```python
from build123d import *

# Parameters (mm, degrees)
BOSS_EXTRUDE1_DEPTH = 6.35
SKETCH2_R           = 2.8575
SKETCH2_W           = 7.62
SKETCH2_H           = 6.5024
SKETCH2_W_2         = 13.97
SKETCH2_H_2         = 3.81
CUT_EXTRUDE1_DEPTH  = 7.35
SKETCH3_W           = 5.334
SKETCH3_H           = 5.08
CUT_EXTRUDE2_DEPTH  = 13.97
SKETCH4_W           = 24.13
SKETCH4_H           = 11.681664872
CUT_EXTRUDE3_DEPTH  = 2.54
FILLET1_R           = 1.5875


with BuildPart() as part:
    # Sketch1 → Boss-Extrude1 (new body)
    with BuildSketch(Plane(origin=(0, 0, 0), x_dir=(0, 0, -1), z_dir=(1, 0, 0))):
        with BuildLine():
            Line((0, 2.54), (0, 14.474335183))
            Line((0, 14.474335183), (38.205942443, 14.474335183))
            ThreePointArc((38.205942443, 14.474335183), (39.475942443, 14.134039708), (40.405646968, 13.204335183))
            Line((40.405646968, 13.204335183), (41.796677285, 10.795))
            ThreePointArc((41.796677285, 10.795), (42.72638181, 9.865295474), (43.99638181, 9.525))
            Line((43.99638181, 9.525), (70.840761314, 9.525))
            Line((70.840761314, 9.525), (66.074734842, 1.27))
            ThreePointArc((66.074734842, 1.27), (65.145030316, 0.340295474), (63.875030316, 0))
            Line((63.875030316, 0), (2.54, 0))
            ThreePointArc((2.54, 0), (0.743948776, 0.743948776), (0, 2.54))
        make_face()
    extrude(amount=BOSS_EXTRUDE1_DEPTH)

    # Sketch2 → Cut-Extrude1 (cut, through all)
    with BuildSketch(Plane(origin=(6.35, 0, 0), x_dir=(0, 0, -1), z_dir=(1, 0, 0))):
        with Locations((59.69, 4.7625)):
            Circle(SKETCH2_R)
        with Locations((46.355, 4.7625)):
            Rectangle(SKETCH2_W, SKETCH2_H)
        with Locations((22.3393, 1.905)):
            Rectangle(SKETCH2_W_2, SKETCH2_H_2)
    extrude(amount=-CUT_EXTRUDE1_DEPTH, mode=Mode.SUBTRACT)

    # Sketch3 → Cut-Extrude2 (cut)
    with BuildSketch(Plane.XY.offset(-29.3243)):
        with Locations((2.667, 6.35)):
            Rectangle(SKETCH3_W, SKETCH3_H)
    extrude(amount=CUT_EXTRUDE2_DEPTH, mode=Mode.SUBTRACT)

    # Sketch4 → Cut-Extrude3 (cut)
    with BuildSketch(Plane(origin=(0, 0, 0), x_dir=(0, 0, -1), z_dir=(1, 0, 0))):
        with Locations((21.0693, 5.840832436)):
            Rectangle(SKETCH4_W, SKETCH4_H)
    extrude(amount=CUT_EXTRUDE3_DEPTH, mode=Mode.SUBTRACT)

    # Fillet1
    fillet1_edges = [part.edges().sort_by_distance(p)[0] for p in [
        (2.54, 8.89, -22.3393),
        (2.54, 4.445, -15.3543),
        (2.54, 4.445, -29.3243),
        (0, 5.840832436, -9.0043),
        (0, 5.840832436, -33.1343),
        (0, 11.681664872, -21.0693),
    ]]
    fillet(fillet1_edges, radius=FILLET1_R)


solid = part.part
```
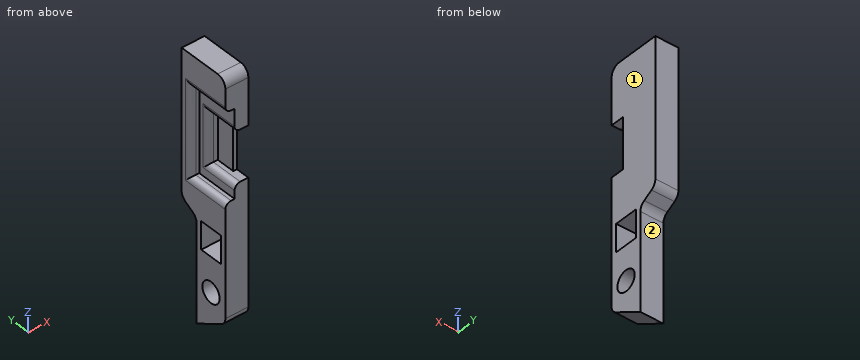
Geometry: final body of the model. Coordinates: model frame, mm. Face numbers are marked on the shaded views. A direction names the side the tool comes from. Coordinates: 2 decimals unless noted, no trailing zeros. Write each loop counter-clockwise with the first axis right and the second up, starting at its lowest first coordinate (ties: lowest second). Pieces come first, ordered by that corner, then holes. Notation, with made-up numbers: M -10.5,74 L -4.5,74 A21 cw -4.5,98 Z; hole C -25,-6 d5. An arc over 180 degrees is marked long. Answer as CSV lines item,"result". Start each with the question number.
Q1. Cut plane C-C on y = 6.25. Count the separate pieces of the cut face and the enclosed holes in it, then the cut area to 3 significant figures.
Q2. Reachability of the marked faces 1 and 2 from +Z, -Z, +X, -X, +Y, -Y: full face, straight path, thin tool, end or side. Return the list, or none.
Q3. Line query: line 1 (Y direction, x = 2.75, z = -59.69) (3 decimals); line 2 (Y direction, x = 1.5, z = -44) (3 decimals); line 3 (Z direction, x = 0.75, y = 7.25) (3 decimals). Output: solid intervals per line, ascending. Write a range as from..to.
Q4. Pin query (flat end, axial travel): P1, Ø0.8, axis at x = 2, z = -15.5, coming from the -Y side; P2, Ø5.5, axis at y = 5.5, z = -24.5, coming from the -X side; P3, Ø0.6, axis at x = 5, z = -21, coming from the -Y side. Return the tip coordinate at first contact, or that it passes through.
Q5. Cut plane A-A on z = -59.69. Return the cut outline in (x, y) (3 decimals).
Findings below:
1,separate pieces,"3"
1,enclosed holes,"0"
1,area,"256 mm2"
2,face 1,"+Z, -Z, +X, +Y, -Y"
2,face 2,"-Z, +X, -X, +Y"
3,line 1,"y = 0..1.905, 7.62..9.525"
3,line 2,"y = 0..1.511, 8.014..9.525"
3,line 3,"z = -69.527..-61.096, -58.284..-50.165, -42.545..-33.373, -8.765..0"
4,P1,"stops at y = 11.68"
4,P2,"stops at x = 5.33"
4,P3,"stops at y = 8.89"
5,outline,"M 0,0 L 6.35,0 L 6.35,1.905 L 0,1.905 Z; M 0,7.62 L 6.35,7.62 L 6.35,9.525 L 0,9.525 Z"
